```python
from build123d import *

# Parameters (mm, degrees)
SKETCH1_W           = 280
SKETCH1_H           = 140
BOSS_EXTRUDE1_DEPTH = 10
SKETCH2_R           = 9.5
CUT_EXTRUDE1_DEPTH  = 10
FILLET1_R           = 10


with BuildPart() as part:
    # Sketch1 → Boss-Extrude1 (new body)
    with BuildSketch(Plane(origin=(0, 0, 0), x_dir=(1, 0, 0), z_dir=(0, 1, 0))):
        Rectangle(SKETCH1_W, SKETCH1_H)
    extrude(amount=BOSS_EXTRUDE1_DEPTH)

    # Sketch2 → Cut-Extrude1 (cut)
    with BuildSketch(Plane(origin=(0, 10, 0), x_dir=(1, 0, 0), z_dir=(0, 1, 0))):
        with Locations(Location((-90, 0, 0), (0, 0, 270))):
            Circle(SKETCH2_R)
        with Locations(Location((0, 0, 0), (0, 0, 270))):
            Circle(SKETCH2_R)
    cut_extrude1 = extrude(amount=-CUT_EXTRUDE1_DEPTH, mode=Mode.SUBTRACT)

    # Mirror1: Cut-Extrude1 across plane
    add(cut_extrude1.mirror(Plane(origin=(0, 0, 0), x_dir=(0, 0, 1), z_dir=(1, 0, 0))), mode=Mode.SUBTRACT)

    # Fillet1
    fillet1_edges = [part.edges().sort_by_distance(p)[0] for p in [
        (140, 5, 70),
        (-140, 5, 70),
    ]]
    fillet(fillet1_edges, radius=FILLET1_R)


solid = part.part
```
Check sheet for the modelled part. Datum: model origin and axes. Units: mm. Round coordinates to 2 decimals unless told otherwise and drop trailing zeros. Loops run counter-clockwise (first coordinate to the right, second up) from the corner with the lowest first, then second, coordinate; pieces in that order, holes last. Notation, with made-up numbers: (40.5, 76) - (53.5, 76) arc R21 cw to (53.5, 100) - close; hole circle Ø10 at (-8.5, 72). An arc over 180 degrees is marked (long way). Answer as a JSON object with one key per item and string values. Group by question number.
Q1. Mould release check, pull along Z, two halves, no side actions. Record for faces 1 (the face through (140, 5, -4)), 2 (the face through (-5.78, 5.07, -7.54)), 3 (the face through (-137.15, 5.07, 66.99)): released by +Z, released by -Z, zero draft, split by the parting line, or undercut.
Q2. Sectioned sample at A-A, the plane z = 0. Enter the section's corners in (x, y), plus the area to 3 significant figures.
Q3. Scan lines: line 1 along X through (y, z) = (5.5, 0); line 2 along Z through (x, y) = (-89.5, 2.25); line 3 along X through (y, z) = (0.75, 61). Record each from-to range of solid material in increasing order. Write a range as [from, to].
Q4. Gauge pin test, flat ends, axial feed: P1, Ø4, axis at x = -103.5, z = 9, coming from the -Y side; P2, Ø11.5, axis at x = 0, z = 0, coming from the -Y side. Record the tip position at first contact, or that the pin passes through.
Q5. Sectioned sample at B-B, the plane x = 90. Enter the section's corners in (y, z).
Q6. Sectioned sample at C-C, the plane y = 5. Enter the section's corners in (x, z).
Solution:
{
 "1": {"face 1": "zero draft", "face 2": "undercut", "face 3": "released by +Z"},
 "2": {"outline": "(-140, 0) - (-99.5, 0) - (-99.5, 10) - (-140, 10) - close; (-80.5, 0) - (-9.5, 0) - (-9.5, 10) - (-80.5, 10) - close; (9.5, 0) - (80.5, 0) - (80.5, 10) - (9.5, 10) - close; (99.5, 0) - (140, 0) - (140, 10) - (99.5, 10) - close", "area": "2,230 mm²"},
 "3": {"line 1": "x = [-140, -99.5], [-80.5, -9.5], [9.5, 80.5], [99.5, 140]", "line 2": "z = [-70, -9.49], [9.49, 70]", "line 3": "x = [-139.95, 139.95]"},
 "4": {"P1": "stops at y = 0", "P2": "passes through"},
 "5": {"outline": "(0, -70) - (10, -70) - (10, -9.5) - (0, -9.5) - close; (0, 9.5) - (10, 9.5) - (10, 70) - (0, 70) - close"},
 "6": {"outline": "(-140, -70) - (140, -70) - (140, 60) arc R10 ccw to (130, 70) - (-130, 70) arc R10 ccw to (-140, 60) - close; hole circle Ø19 at (-90, 0); hole circle Ø19 at (0, 0); hole circle Ø19 at (90, 0)"}
}
